```python
from build123d import *

# Parameters (mm, degrees)
SKETCH_1_W          = 28
SKETCH_1_H          = 30
EXTRUDE_1_DEPTH     = 5
SKETCH_2_W          = 28
SKETCH_2_H          = 5
EXTRUDE_2_DEPTH     = 15
SKETCH_3_R          = 1.7
CUT_EXTRUDE_1_DEPTH = 5
SKETCH_4_R          = 1.7
CUT_EXTRUDE_2_DEPTH = 5
FILLET_1_SIZE       = 9
FILLET_1_SIZE_2     = 4


with BuildPart() as part:
    # 草图1 → 凸台-拉伸1 (new body)
    with BuildSketch(Plane(origin=(0, 0, 0), x_dir=(1, 0, 0), z_dir=(0, 1, 0))):
        with Locations((14, -15)):
            Rectangle(SKETCH_1_W, SKETCH_1_H)
    extrude(amount=EXTRUDE_1_DEPTH)

    # 草图2 → 凸台-拉伸2 (add)
    with BuildSketch(Plane(origin=(0, 5, 0), x_dir=(1, 0, 0), z_dir=(0, 1, 0))):
        with Locations((14, -2.5)):
            Rectangle(SKETCH_2_W, SKETCH_2_H)
    extrude(amount=EXTRUDE_2_DEPTH)

    # 草图3 → 切除-拉伸1 (cut)
    with BuildSketch(Plane(origin=(0, 5, 0), x_dir=(1, 0, 0), z_dir=(0, 1, 0))):
        with Locations(Location((4, -23.725, 0), (0, 0, 270))):
            Circle(SKETCH_3_R)
        with Locations(Location((24, -23.725, 0), (0, 0, 90))):
            Circle(SKETCH_3_R)
    extrude(amount=-CUT_EXTRUDE_1_DEPTH, mode=Mode.SUBTRACT)

    # 草图4 → 切除-拉伸2 (cut)
    with BuildSketch(Plane.XY.offset(5)):
        with Locations((5, 15)):
            Circle(SKETCH_4_R)
        with Locations(Location((23, 15, 0), (0, 0, 180))):
            Circle(SKETCH_4_R)
    extrude(amount=-CUT_EXTRUDE_2_DEPTH, mode=Mode.SUBTRACT)

    # 圆角1
    # an asymmetric fillet: 9, 4 mm, written as the material it adds along each edge
    with BuildSketch(Plane(origin=(28, 5, 5), x_dir=(0, 0, 1), z_dir=(-1, 0, 0))) as fillet_1_piece_1:
        with BuildLine():
            Bezier((FILLET_1_SIZE, 0), (0, 0), (0, FILLET_1_SIZE_2), weights=[1, 0.707106781, 1])
            Line((0, FILLET_1_SIZE_2), (0, 0))
            Line((0, 0), (FILLET_1_SIZE, 0))
        make_face()
    extrude(amount=28)


solid = part.part
```
Here's how the part is built. I have some questions about the finished solid (model axes, mm). A direction names the side the tool comes from. Give positions to 0.01 mm unless a question says otherwise; leave off trailing zeros. Write each loop counter-clockwise with the first axis right and the second up, starting at its lowest first coordinate (ties: lowest second). Pieces come first, ordered by that corner, then holes. Notation, with made-up numbers: (55.25, 39.5) -> (96.25, 39.5) arc R26 ccw to (96.25, 70.5) -> close; hole circle Ø4 at (50.25, 88.5). An arc over 180 degrees is marked (long way). Write each question's results on one line, items separated by ' | '.
Item 1: Suppose I cut it at C-C on z = 15.5. Write out the boundary of the cut face in (x, y).
Output:
outline: (0, 0) -> (28, 0) -> (28, 5) -> (0, 5) -> close
Item 2: For pin 1 Ø8 at (x, z) = (11.5, 25) entering from +Y; pin 2 Ø5 at (x, y) = (23.5, 15.5) entering from +Z; pin 3 Ø1 at (x, y) = (11.5, 7) entering from +Z; pin 4 Ø3 at (x, y) = (23, 15) entering from +Z, each with a flat end and sliding along its axis, tell me the tip position at first contact or that it passes through.
Output:
pin 1: stops at y = 5 | pin 2: stops at z = 5 | pin 3: stops at z = 6.97 | pin 4: passes through
Item 3: Suppose I cut it at A-A on y = 15. Write out the boundary of the cut face in (x, z).
Output:
outline: (0, 0) -> (3.3, 0) -> (3.3, 5) -> (0, 5) -> close; (6.7, 0) -> (21.3, 0) -> (21.3, 5) -> (6.7, 5) -> close; (24.7, 0) -> (28, 0) -> (28, 5) -> (24.7, 5) -> close
Item 4: Suppose I cut it at D-D on x = 23. Give the number of separate pieces and of enclosed holes in the cut face, plus the area to 3 significant figures.
Output:
separate pieces: 3 | enclosed holes: 0 | area: 202 mm^2
Item 5: On a 3-axis mill with a long thin cutter (end or side, diameter ignored), from which of +Z, -Z, +X, -X, +Y, -Y can I reach the whole of each face in a straight line? I mean faces 1 (the face through (5.8, 13.5, 2.5)), 2 (the face through (14, 5, 22)). Say none if no direction works.
Output:
face 1: +Z, -Z | face 2: +Z, +X, -X, +Y
Item 6: We'd pull the mould along X, two halves only. Please class faces 3 (the face through (28, 5.7, 8.1)), 4 (the face through (21.43, 15.65, 2.54)), 5 (the face through (14, 14, 5)): pulls with the +X half, pulls with the -X half, needs draft (parallel to the pull), parting line crosses it, or undercut.
Output:
face 3: pulls with the +X half | face 4: undercut | face 5: needs draft
Item 7: If I drill on L1, parallel to Y at x = 23, z = 2.6; L2, parallel to Z at x = 24, y = 2.9 (3 decimals); L3, parallel to Y at x = 23.25, z = 18, over which ranges is the centre line in solid material (lowest first)?
Output:
L1: y = 0 to 13.3, 16.7 to 20 | L2: z = 0 to 22.025, 25.425 to 30 | L3: y = 0 to 5
Item 8: Suppose I cut it at B-B on y = 4.5. Write out the boundary of the cut face in (x, z) (3 decimals).
Output:
outline: (0, 0) -> (28, 0) -> (28, 30) -> (0, 30) -> close; hole circle Ø3.4 at (4, 23.725); hole circle Ø3.4 at (24, 23.725)
